Source: three-view drawing plus pictorial views. Frame: mm from the lowest corner of the part. Give positions to 0.01 mm unless a question says otherwise; leave off trailing zeros. Order: outer loops, then holes, each group sorted by start corner. A loop starts at its lowest first (then second) coordinate and runs counter-clockwise, first axis right, second up.
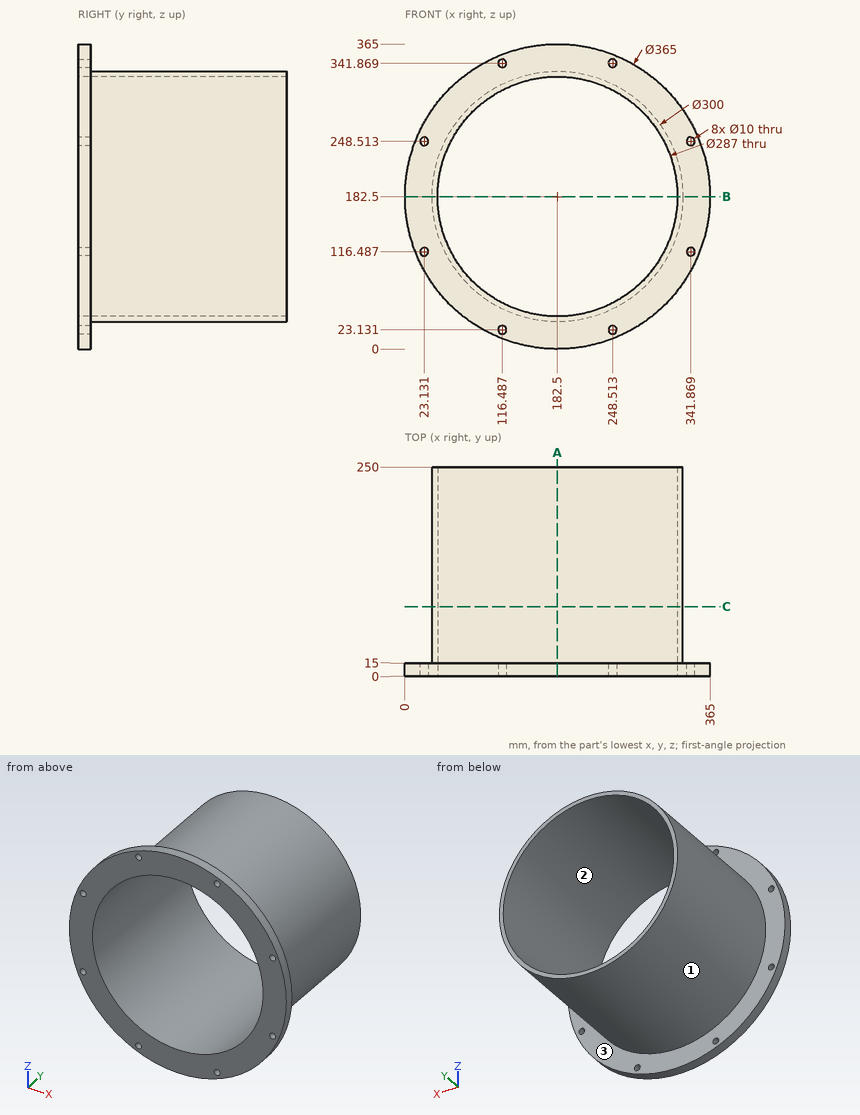
1) First-contact query: pin 1 Ø8 at (x, y) = (82, 148.5) entering from -Z; pin 2 Ø8 at (x, z) = (221, 42) entering from -Y; pin 3 Ø5 at (x, y) = (286, 209) entering from -Z; pin 4 Ø13 at (x, z) = (116.49, 341.87) entering from +Y. Flat tips, straight axial feed; report the tip coordinate or a pass-through.
Checks:
pin 1: stops at z = 67.66
pin 2: stops at y = 0
pin 3: stops at z = 71.6
pin 4: stops at y = 15
2) Section query B-B on z = 182.5. Output: boundary loops of the cut face in (x, y).
Checks:
outline: (0, 0) - (39, 0) - (39, 250) - (32.5, 250) - (32.5, 15) - (0, 15) - close; (326, 0) - (365, 0) - (365, 15) - (332.5, 15) - (332.5, 250) - (326, 250) - close
3) Section query C-C on y = 83. Output: boundary loops of the cut face in (x, z), and give its area (3 significant figures).
Checks:
outline: circle Ø300 at (182.5, 182.5); hole circle Ø287 at (182.5, 182.5)
area: 5,990 mm2
4) Pull-direction query (X, two-part tool) for the marked faces 1, 2 and 3; classes: +X half, -X half, draft (parallel to the pull), parting line (faces both ways), or undercut.
Checks:
face 1: parting line
face 2: undercut
face 3: draft
5) Ray query, L1, parallel to Y at x = 260, z = 327; L2, parallel to Z at x = 150.5, y = 135; L3, parallel to Z at x = 87, y = 144. Return the intervals inside material, ascending.
Checks:
L1: y = 0 to 15
L2: z = 35.95 to 42.61, 322.39 to 329.05
L3: z = 66.83 to 75.39, 289.61 to 298.17
6) Section query A-A on x = 182.5. Output: boundary loops of the cut face in (y, z).
Checks:
outline: (0, 0) - (15, 0) - (15, 32.5) - (250, 32.5) - (250, 39) - (0, 39) - close; (0, 326) - (250, 326) - (250, 332.5) - (15, 332.5) - (15, 365) - (0, 365) - close
